Can you work these out from the model? Positions are in its coordinate system, mm. A direction names the side the tool comes from. Give positions to 0.01 mm unless a question says otherwise; leave off trailing zeros. Order: outer loops, then holes, each group sorted by start corner. A loop starts at its lowest first (then second) coordinate and runs counter-clockwise, first axis right, second up.
Item 1: I want a section at C-C, the plane x = -4. Write out the boundary of the cut face in (y, z), then the cut area to 3 significant figures.
Item 2: If we mould it in two halves opening along X, with no side actions, what happens to faces 1 (the flat face through (0, 7, 3)), 2 (the cylindrical face through (8.45, 31.71, 8.49)), 3 (the flat face through (4, 32, -1))? For each: +X half, -X half, draft (parallel to the pull), parting line (faces both ways), or undercut.
Item 3: I'm going to push flat-ended pins straight in: pin 1 Ø5 at (y, z) = (46, 5) entering from -X; pin 2 Ø16 at (x, y) = (-3, 1.5) entering from -Z; pin 3 Ø16 at (x, y) = (0, 0) entering from -Z. Where does each tip first touch, or does it pass through?
Item 4: I want a section at B-B, the plane z = 6.75. Write out the boundary of the cut face in (x, y).
Item 5: Which directions (+Z, -Z, +X, -X, +Y, -Y) give clear straight access to the entire face, cutting with the end or side of a thin tool? Please do faces 4 (the cylindrical face through (-2.17, -9.76, 6.48)), 5 (the cylindrical face through (0, 65, 3)), 6 (the cylindrical face through (-8.45, 31.71, -0.51)).
Item 6: I want a section at A-A, the plane y = 0. Write out the boundary of the cut face in (x, z).
Item 7: If I drill on line 1 along Y through (x, z) = (0, 2); line 2 along Y through (x, z) = (0, 4.35); line 3 along X through (y, z) = (0, 6.7), over which ranges is the centre line in solid material (lowest first)?
Item 8: I want a section at D-D, the plane y = 22.5. Write out the boundary of the cut face in (x, z), then the cut area to 3 significant figures.
```python
from build123d import *

# Parameters (mm, degrees)
SKETCH_1_R               = 6
EXTRUDE_2_DEPTH          = 8
CUT_EXTRUDE_START        = -3
SKETCH_2_R               = 10
SKETCH_2_R_2             = 6
CUT_EXTRUDE_1_DEPTH      = 3
SKETCH_3_R               = 10
SKETCH_3_R_2             = 6
CUT_EXTRUDE_2_DEPTH      = 3
SKETCH_5_R               = 0.5
CUT_EXTRUDE_3_DEPTH      = 68.788273322
SKETCH_6_R               = 10
CUT_EXTRUDE_4_DEPTH      = 68.788273322
EXTRUDE_START            = 1
SKETCH_7_R               = 12.5
SKETCH_7_R_2             = 10
EXTRUDE_3_DEPTH          = 1
SKETCH_8_R               = 12.5
SKETCH_8_R_2             = 10
EXTRUDE_4_DEPTH          = 1
CUT_EXTRUDE_5_REACH      = 86.815
CUT_EXTRUDE_5_END_RADIUS = 0.5
SKETCH_10_R              = 0.5


with BuildPart() as part:
    # 草图1 → 凸台-拉伸2 (new body)
    with BuildSketch(Plane.XY):
        with BuildLine():
            ThreePointArc((4.850754193, 61.212511345), (0, 65), (-4.850754193, 61.212511345))
            ThreePointArc((-4.850754193, 61.212511345), (-11.55450868, 32.234679821), (-17.234135678, 3.038843109))
            ThreePointArc((-17.234135678, 3.038843109), (0, -17.5), (17.234135678, 3.038843109))
            ThreePointArc((17.234135678, 3.038843109), (11.55450868, 32.234679821), (4.850754193, 61.212511345))
        make_face()
        Circle(SKETCH_1_R, mode=Mode.SUBTRACT)
    extrude(amount=EXTRUDE_2_DEPTH)

    # 草图2 → 切除-拉伸1 (cut)
    with BuildSketch(Plane.XY.offset(8).offset(CUT_EXTRUDE_START)):
        Circle(SKETCH_2_R)
        Circle(SKETCH_2_R_2, mode=Mode.SUBTRACT)
    extrude(amount=CUT_EXTRUDE_1_DEPTH, mode=Mode.SUBTRACT)

    # 草图3 → 切除-拉伸2 (cut)
    with BuildSketch(Plane(origin=(0, 0, 0), x_dir=(-1, 0, 0), z_dir=(0, 0, -1))):
        with Locations(Location((0, 0, 0), (0, 0, 180))):
            Circle(SKETCH_3_R)
        Circle(SKETCH_3_R_2, mode=Mode.SUBTRACT)
    extrude(amount=-CUT_EXTRUDE_2_DEPTH, mode=Mode.SUBTRACT)

    # 草图5 → 切除-拉伸3 (cut, through all)
    with BuildSketch(Plane(origin=(0, 0, 0), x_dir=(-1, 0, 0), z_dir=(0, 0, -1))):
        with Locations((0, 60)):
            Circle(SKETCH_5_R)
    extrude(amount=-CUT_EXTRUDE_3_DEPTH, mode=Mode.SUBTRACT)

    # 草图6 → 切除-拉伸4 (cut, through all)
    with BuildSketch(Plane(origin=(0, 0, 0), x_dir=(-1, 0, 0), z_dir=(0, 0, -1))):
        with Locations((0, 22.5)):
            Circle(SKETCH_6_R)
    extrude(amount=-CUT_EXTRUDE_4_DEPTH, mode=Mode.SUBTRACT)

    # 草图7 → 凸台-拉伸3 (add)
    with BuildSketch(Plane(origin=(0, 0, 0), x_dir=(-1, 0, 0), z_dir=(0, 0, -1)).offset(EXTRUDE_START)):
        with Locations(Location((0, 22.5, 0), (0, 0, 270))):
            Circle(SKETCH_7_R)
        with Locations((0, 22.5)):
            Circle(SKETCH_7_R_2, mode=Mode.SUBTRACT)
    extrude(amount=-EXTRUDE_3_DEPTH)

    # 草图8 → 凸台-拉伸4 (add)
    with BuildSketch(Plane.XY.offset(8)):
        with Locations(Location((0, 22.5, 0), (0, 0, 270))):
            Circle(SKETCH_8_R)
        with Locations(Location((0, 22.5, 0), (0, 0, 180))):
            Circle(SKETCH_8_R_2, mode=Mode.SUBTRACT)
    extrude(amount=EXTRUDE_4_DEPTH)

    # 切除-拉伸5: up to this cylinder (the profile starts outside it)
    cut_extrude_5_end = Plane(origin=(0, 60, 4), z_dir=(0, 0, -1)) * Cylinder(CUT_EXTRUDE_5_END_RADIUS, 175.63, mode=Mode.PRIVATE)
    # 草图10 → 切除-拉伸5 (cut, up to the surface)
    with BuildSketch(Plane(origin=(0, 65, 0), x_dir=(1, 0, 0), z_dir=(0, 1, 0)), mode=Mode.PRIVATE) as cut_extrude_5_sk1:
        with Locations(Location((0, -4, 0), (0, 0, 180))):
            Circle(SKETCH_10_R)
    cut_extrude_5_tool1 = extrude(cut_extrude_5_sk1.sketch, amount=-CUT_EXTRUDE_5_REACH, mode=Mode.PRIVATE) - cut_extrude_5_end
    add(cut_extrude_5_tool1.solids().sort_by_distance((0, 65, 4))[0], mode=Mode.SUBTRACT)


solid = part.part
```
Results list:
1. outline: (-17.04, 0) - (-9.17, 0) - (-9.17, 3) - (-4.47, 3) - (-4.47, 5) - (-9.17, 5) - (-9.17, 8) - (-17.04, 8) - close; (4.47, 3) - (9.17, 3) - (9.17, 0) - (10.66, 0) - (10.66, -1) - (13.33, -1) - (13.33, 9) - (10.66, 9) - (10.66, 8) - (9.17, 8) - (9.17, 5) - (4.47, 5) - close; (31.67, -1) - (34.34, -1) - (34.34, 0) - (63, 0) - (63, 8) - (34.34, 8) - (34.34, 9) - (31.67, 9) - close
1. area: 376 mm2
2. face 1: undercut
2. face 2: parting line
2. face 3: draft
3. pin 1: stops at x = -9.08
3. pin 2: stops at z = 0
3. pin 3: stops at z = 3
4. outline: (-17.23, 3.04) arc R17.5 ccw (long way) to (17.23, 3.04) arc R844.88 ccw to (4.85, 61.21) arc R5 ccw to (-4.85, 61.21) arc R844.88 ccw to start; hole circle Ø20 at (0, 0); hole circle Ø20 at (0, 22.5); hole circle Ø1 at (0, 60)
5. face 4: +Z
5. face 5: +Z, -Z, +Y
5. face 6: -Z
6. outline: (-17.5, 0) - (-10, 0) - (-10, 3) - (-6, 3) - (-6, 5) - (-10, 5) - (-10, 8) - (-17.5, 8) - close; (6, 3) - (10, 3) - (10, 0) - (17.5, 0) - (17.5, 8) - (10, 8) - (10, 5) - (6, 5) - close
7. line 1: y = -17.5 to -10, 10 to 12.5, 32.5 to 59.5, 60.5 to 65
7. line 2: y = -17.5 to -6, 6 to 12.5, 32.5 to 59.5
7. line 3: x = -17.5 to -10, 10 to 17.5
8. outline: (-13.57, 0) - (-12.5, 0) - (-12.5, -1) - (-10, -1) - (-10, 9) - (-12.5, 9) - (-12.5, 8) - (-13.57, 8) - close; (10, -1) - (12.5, -1) - (12.5, 0) - (13.57, 0) - (13.57, 8) - (12.5, 8) - (12.5, 9) - (10, 9) - close
8. area: 67.1 mm2
